The listing builds one solid part. Answer for the finished solid, in the listing's coordinates (mm). Coordinates: 2 decimals unless noted, no trailing zeros. Order: outer loops, then holes, each group sorted by start corner. A loop starts at its lowest first (then second) coordinate and runs counter-clockwise, first axis right, second up. Notation, with made-up numbers: (22, 86.25) -> (37, 86.25) arc R15 ccw to (37, 109.25) -> close; hole circle Ø4 at (87, -1). An arc over 180 degrees is marked (long way). Write each question's results on one line, items separated by ' | '. Start each with the question number.
(1) The part is cut by section D-D, the plane x = -42. Give the vertices of the cut face in (y, z).
(2) Given pin 1 (0.5 mm diameter, centred on y = 13.5, z = 0.5, fed in from +X); pin 2 (0.5 mm diameter, centred on x = 7, z = 0.5, fed in from +Y); pin 3 (0.5 mm diameter, centred on y = 34.5, z = 0.5, fed in from -X); pin 4 (1 mm diameter, centred on x = 0, y = -15, fed in from -Z), each flat-ended and moving along its own axis, determine where each tip first touches the part or whether it passes through.
(3) The part is cut by section B-B, the plane y = 21.75. Give the vertices of the cut face in (x, z).
(4) Straight lines are drawn through the part: L1, parallel to Y at x = -35, z = 0.8; L2, parallel to Y at x = 1.43, z = 0.85; L3, parallel to X at y = 21, z = 0.3. For each, find the intervals that lie inside material, in ascending order.
(5) Determine the mould class of faces 1 (the face through (-49.99, -0.93, 0.49)), 2 (the face through (-12, 1, 1)), 3 (the face through (-35.99, 7.14, 0.51)) for opening direction Y: +Y half, -Y half, draft (parallel to the pull), parting line (faces both ways), or undercut.
(6) The part is cut by section A-A, the plane x = 18.57. Give the vertices of the cut face in (y, z).
(7) The part is cut by section C-C, the plane z = 0.85. Count the separate pieces of the cut face and the enclosed holes in it, then the cut area to 3 significant figures.
Autodesk Inventor part; units mm, degrees
ref_plane "YZ Plane" through (0, 0, 0) normal (1, 0, 0) x (0, 1, 0)
ref_plane "XZ Plane" through (0, 0, 0) normal (0, 1, 0) x (-1, 0, 0)
ref_plane "XY Plane" through (0, 0, 0) normal (0, 0, 1) x (1, 0, 0)
sketch "Sketch1" plane through (0, 0, 0) normal (0, 0, 1) x (1, 0, 0)
  circle A0 centre (0, 0) radius 50
  dimension "d0" = 100
extrude "Extrusion1" add sketch "Sketch1" along normal blind 1
sketch "Sketch3" plane through (0, 0, 1) normal (0, 0, 1) x (1, 0, 0)
  circle A0 centre (0, 0) radius 50 construction
  line L0 (50, 0) -> (-50, 0)
  line L1 (10, 28) -> (-12, 28)
  line L2 (10, 28) -> (32, 28)
  line L3 (32, 28) -> (32, 38.4187)
  line L4 (-12, 28) -> (-12, 48.5386)
  line L5 (0, 0) -> (0, 50) construction
  arc A1 (32, 38.4187) -> (-12, 48.5386) centre (0, 0) ccw
  line L6 (32, -38.4187) -> (32, -28)
  line L7 (32, -28) -> (10, -28)
  line L8 (10, -28) -> (-12, -28)
  line L9 (-12, -28) -> (-12, -48.5386)
  line L10 (0, 0) -> (0, -50) construction
  arc A2 (-12, -48.5386) -> (32, -38.4187) centre (0, 0) ccw
  arc A3 (32, 38.4187) -> (-12, 48.5386) centre (0, 0) ccw
  dimension "d18" = 100
  dimension "d19" = 44
  dimension "d21" = 22
  dimension "d22" = 10
  dimension "d23" = 44
  dimension "d24" = 22
  dimension "d25" = 10
extrude "Extrusion4" cut sketch "Sketch3" against normal through all
sketch "Sketch4" plane through (0, 0, 1) normal (0, 0, 1) x (1, 0, 0)
  line L0 (0, 0) -> (10, 0)
  line L1 (10, 0) -> (10, 12)
  line L2 (10, 0) -> (10, -12)
  line L3 (-0.75, -15.75) -> (20.75, -15.75)
  line L4 (20.75, -15.75) -> (20.75, -8.25)
  line L5 (20.75, -8.25) -> (-0.75, -8.25)
  line L6 (-0.75, -8.25) -> (-0.75, -15.75)
  line L7 (-0.75, -15.75) -> (20.75, -8.25) construction
  line L8 (20.75, -15.75) -> (-0.75, -8.25) construction
  line L9 (-0.75, 8.25) -> (20.75, 8.25)
  line L10 (20.75, 8.25) -> (20.75, 15.75)
  line L11 (20.75, 15.75) -> (-0.75, 15.75)
  line L12 (-0.75, 15.75) -> (-0.75, 8.25)
  line L13 (-0.75, 8.25) -> (20.75, 15.75) construction
  line L14 (20.75, 8.25) -> (-0.75, 15.75) construction
  dimension "d28" = 10
  dimension "d29" = 12
  dimension "d30" = 12
  dimension "d31" = 21.5
  dimension "d32" = 7.5
  dimension "d33" = 21.5
  dimension "d34" = 7.5
extrude "Extrusion5" cut sketch "Sketch4" against normal through all
sketch "Sketch5" plane through (0, 0, 1) normal (0, 0, 1) x (1, 0, 0)
  circle A0 centre (0, 0) radius 5
  dimension "d37" = 10
extrude "Extrusion6" cut sketch "Sketch5" against normal through all
sketch "Sketch6" plane through (0, 0, 1) normal (0, 0, 1) x (1, 0, 0)
  line L0 (20.75, -15.75) -> (-0.75, -15.75)
  line L1 (-0.75, 15.75) -> (20.75, 15.75)
  line L2 (20.75, 15.75) -> (-0.75, 15.75)
  line L3 (10, 15.75) -> (10, 21.75)
  line L4 (10, -15.75) -> (10, -21.75)
  line L5 (1.43, 21.75) -> (18.57, 21.75)
  line L6 (1.43, -21.75) -> (18.57, -21.75)
  circle A0 centre (1.43, 21.75) radius 1.25
  circle A1 centre (18.57, 21.75) radius 1.25
  circle A2 centre (1.43, -21.75) radius 1.25
  circle A3 centre (18.57, -21.75) radius 1.25
  point P0 (0, 0)
  dimension "d40" = 6
  dimension "d41" = 6
  dimension "d42" = 17.14
  dimension "d43" = 17.14
  dimension "d44" = 2.5
  dimension "d45" = 2.5
  dimension "d46" = 2.5
  dimension "d47" = 2.5
extrude "Extrusion7" cut sketch "Sketch6" against normal through all
sketch "Sketch7" plane through (0, 0, 1) normal (0, 0, 1) x (1, 0, 0)
  line L0 (0, 0) -> (-35, 0)
  line L1 (-35, -7.9) -> (-35, 7.9)
  circle A0 centre (-35, -7.9) radius 1.25
  circle A1 centre (-35, 7.9) radius 1.25
  dimension "d50" = 35
  dimension "d51" = 15.8
  dimension "d52" = 2.5
  dimension "d53" = 2.5
extrude "Extrusion8" cut sketch "Sketch7" against normal through all
sketch "Sketch8" plane through (0, 0, 1) normal (0, 0, 1) x (1, 0, 0)
  line L0 (0, 0) -> (-42, 0) construction
  line L1 (0, 0) -> (38, 0) construction
  line L2 (38, 0) -> (38, 18) construction
  line L3 (38, 0) -> (38, -18) construction
  circle A0 centre (-42, 0) radius 1.5
  circle A1 centre (38, 18) radius 1.5
  circle A2 centre (38, -18) radius 1.5
  dimension "d56" = 42
  dimension "d57" = 38
  dimension "d58" = 18
  dimension "d59" = 3
extrude "Extrusion9" cut sketch "Sketch8" against normal through all
equation "\"d23\" = d19"
equation "\"d24\" = d21"
equation "\"d25\" = d22"
equation "\"d28\" = d22"
equation "\"d29\" = d30"
equation "\"d33\" = d31"
equation "\"d34\" = d32"
equation "\"d38\" = d37"
equation "\"d43\" = d42"
properties part number "Base Inferior" material "Glass"
Established:
1) outline: (-27.13, 0) -> (-1.5, 0) -> (-1.5, 1) -> (-27.13, 1) -> close; (1.5, 0) -> (27.13, 0) -> (27.13, 1) -> (1.5, 1) -> close
2) pin 1: stops at x = 48.21 | pin 2: stops at y = 28 | pin 3: stops at x = -36.43 | pin 4: passes through
3) outline: (-45.02, 0) -> (0.18, 0) -> (0.18, 1) -> (-45.02, 1) -> close; (2.68, 0) -> (17.32, 0) -> (17.32, 1) -> (2.68, 1) -> close; (19.82, 0) -> (45.02, 0) -> (45.02, 1) -> (19.82, 1) -> close
4) L1: y = -35.71 to -9.15, -6.65 to 6.65, 9.15 to 35.71 | L2: y = -28 to -23, -20.5 to -15.75, -8.25 to -4.79, 4.79 to 8.25, 15.75 to 20.5, 23 to 28 | L3: x = -45.38 to 0.43, 2.43 to 17.57, 19.57 to 45.38
5) face 1: parting line | face 2: draft | face 3: undercut
6) outline: (-28, 0) -> (-23, 0) -> (-23, 1) -> (-28, 1) -> close; (-20.5, 0) -> (-15.75, 0) -> (-15.75, 1) -> (-20.5, 1) -> close; (-8.25, 0) -> (8.25, 0) -> (8.25, 1) -> (-8.25, 1) -> close; (15.75, 0) -> (20.5, 0) -> (20.5, 1) -> (15.75, 1) -> close; (23, 0) -> (28, 0) -> (28, 1) -> (23, 1) -> close
7) separate pieces: 1 | enclosed holes: 12 | area: 5,710 mm^2
